Study the drawing (mm; zero at the part's minimum x, y, z) and answer. Give positions to 0.01 mm unless a question says otherwise; leave off trailing zeros. Order: outer loops, then holes, each group sorted by start corner. A loop starts at its lowest first (then second) coordinate and runs counter-clockwise, first axis right, second up.
Item 1: A cutting plane is placed at C-C (x = 177). Write down the section's boundary in (y, z), plus the area to 3 significant figures.
Item 2: A cutting plane is placed at B-B (x = 21.5). Write down the section's boundary in (y, z).
Item 3: A cutting plane is placed at A-A (y = 12.7). Write down the section's boundary in (x, z).
Item 4: Find the intervals of material crossed by line 1 along X through (y, z) = (12, 2.15) (1 decimal), in increasing order.
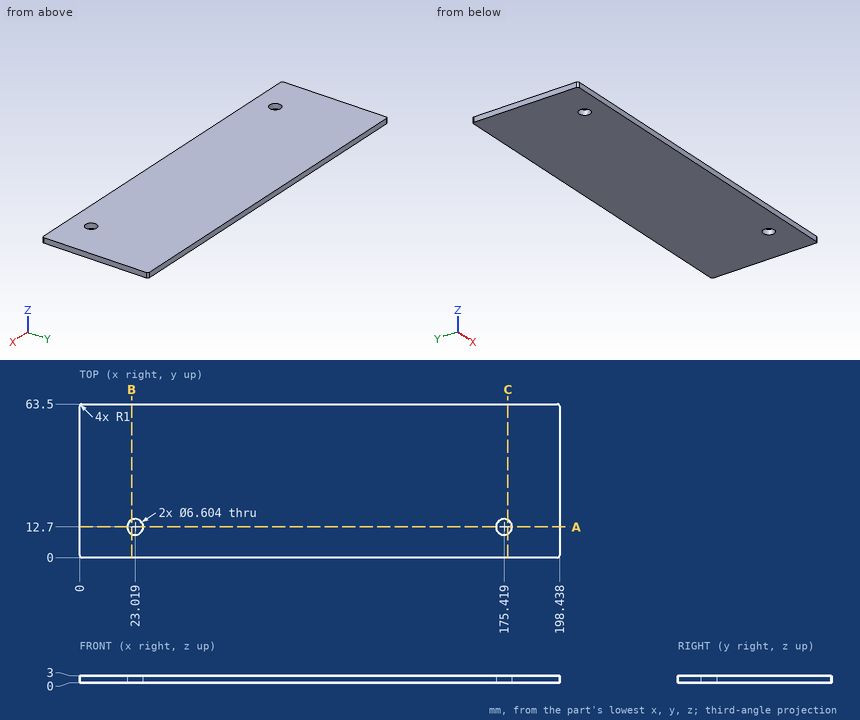
Response values:
1. outline: (0, 0) - (9.8, 0) - (9.8, 3) - (0, 3) - close; (15.6, 0) - (63.5, 0) - (63.5, 3) - (15.6, 3) - close
1. area: 173 mm2
2. outline: (0, 0) - (9.77, 0) - (9.77, 3) - (0, 3) - close; (15.63, 0) - (63.5, 0) - (63.5, 3) - (15.63, 3) - close
3. outline: (0, 0) - (19.72, 0) - (19.72, 3) - (0, 3) - close; (26.32, 0) - (172.12, 0) - (172.12, 3) - (26.32, 3) - close; (178.72, 0) - (198.44, 0) - (198.44, 3) - (178.72, 3) - close
4. line 1: x = 0 to 19.8, 26.2 to 172.2, 178.6 to 198.4
